For this review, take the finished solid that the model builds, in its own axes (mm). A direction names the side the tool comes from. Coordinates: 2 decimals unless noted, no trailing zeros. Order: outer loops, then holes, each group sorted by start corner. A loop starts at its lowest first (then second) coordinate and runs counter-clockwise, first axis right, second up.
Autodesk Fusion 360 part; units mm, degrees
sketch "Sketch1" plane through (0, 0, 0) normal (0, 0, 1) x (1, 0, 0)
  line L0 (8.375, 6.75) -> (-8.375, 6.75)
  line L1 (-8.375, -6.75) -> (8.375, -6.75)
  line L2 (8.375, -6.75) -> (8.375, 6.75)
  line L3 (8.375, 6.75) -> (-8.375, -6.75) construction
  line L4 (-8.375, 6.75) -> (8.375, -6.75) construction
  line L5 (-9, 12.0754) -> (13, 12.0754)
  line L6 (13, 12.0754) -> (13, -12.0754)
  line L7 (13, -12.0754) -> (-9, -12.0754)
  line L8 (-9, -12.0754) -> (-9, 12.0754)
  line L9 (-9, 12.0754) -> (13, -12.0754) construction
  line L10 (13, 12.0754) -> (-9, -12.0754) construction
  line L11 (-8.375, -6.75) -> (-9, -6.75)
  line L12 (-8.375, 6.75) -> (-9, 6.75)
  point P0 (2, 0)
  dimension "d1" = 16.75
  dimension "d2" = 13.5
extrude "Extrude1" add sketch "Sketch1" along normal blind 7
extrude "Extrude2" cut sketch "Sketch1" along normal blind 4.5 and the other way blind -1.5 contours L0 L1 L2 L5 L6 L7 L8 L11 L12
extrude "Extrude3" add 1 faces at (13, 4.0251, 6.1667) along direction (1, 0, 0) blind 2
1. To check wall thickness, follow L1, parallel to Z at x = 2.25, y = 8.75; L2, parallel to Y at x = 3, z = 2.5; L3, parallel to X at y = -1.5, z = 0.75. State the ranges of each line that lie inside material, in increasing order.
Answer below:
L1: z = 0 to 1.5, 4.5 to 7
L2: y = -6.75 to 6.75
L3: x = -9 to 13
2. Take a section at A-A, the plane y = 9. Give the boundary of the cut face in (x, z).
Answer below:
outline: (-9, 0) - (13, 0) - (13, 1.5) - (-9, 1.5) - close; (-9, 4.5) - (15, 4.5) - (15, 7) - (-9, 7) - close
3. Clearance check with flat-ended pins moving along their axes: pin 1 Ø1.6 at (y, z) = (-5, 1) entering from +X; pin 2 Ø0.9 at (x, z) = (-0.5, 3) entering from +Y; pin 3 Ø1 at (y, z) = (-3, 3.5) entering from +X (3 decimals). State where each tip first meets the part, or that it passes through.
Answer below:
pin 1: stops at x = 13
pin 2: stops at y = 6.75
pin 3: stops at x = 8.375
4. Take a section at D-D, the plane z = 3.75. Give the boundary of the cut face in (x, y) (3 decimals).
Answer below:
outline: (-9, -6.75) - (8.375, -6.75) - (8.375, 6.75) - (-9, 6.75) - close
5. Take a section at B-B, the plane x = -5. Give the boundary of the cut face in (y, z), plus the area to 3 significant figures.
Answer below:
outline: (-12.08, 0) - (12.08, 0) - (12.08, 1.5) - (6.75, 1.5) - (6.75, 4.5) - (12.08, 4.5) - (12.08, 7) - (-12.08, 7) - (-12.08, 4.5) - (-6.75, 4.5) - (-6.75, 1.5) - (-12.08, 1.5) - close
area: 137 mm2
6. Take a section at C-C, the plane y = 3.75. Give the boundary of the cut face in (x, z) (3 decimals), plus the area to 3 significant figures.
Answer below:
outline: (-9, 0) - (13, 0) - (13, 1.5) - (8.375, 1.5) - (8.375, 4.5) - (15, 4.5) - (15, 7) - (-9, 7) - close
area: 145 mm2
7. The part is to be moulded in two halves that separate along Z. For faces 5 (the face through (2, 0, 0)), 6 (the face through (8.375, 0, 3)), 7 (the face through (3, 12.075, 6)), say which applies: +Z half, -Z half, draft (parallel to the pull), parting line (faces both ways), or undercut.
Answer below:
face 5: -Z half
face 6: undercut
face 7: draft
8. Machinability: for faces 1 (the face through (13, 0, 1)), 2 (the face through (9, 0, 1.5)), 3 (the face through (0, 6.75, 3)), 4 (the face through (0, -6.75, 3)), which of the approach directions +Z, -Z, +X, -X, +Y, -Y give a long, thin tool a straight path to every point of the face, cutting with its end or side? Answer none if there is none.
Answer below:
face 1: -Z, +X, +Y, -Y
face 2: +X
face 3: +X, -X, +Y
face 4: +X, -X, -Y
